Check sheet for the modelled part. Datum: model origin and axes. Units: mm. A direction names the side the tool comes from. Coordinates: 2 decimals unless noted, no trailing zeros. Loops run counter-clockwise (first coordinate to the right, second up) from the corner with the lowest first, then second, coordinate; pieces in that order, holes last. Notation, with made-up numbers: M 66,56.25 L 110,56.25 A18 ccw 110,86.25 Z; hole C 55.5,58.25 d1. An arc over 180 degrees is marked long. Use CSV: the item, a comma, the result in double quotes. Start each with the question number.
(1) Section check C-C on x = 34.5. Record the cut outline in (y, z).
(2) Set-up check for faces 4 (the flat face through (53, -60, 108)), 5 (the flat face through (39, -63, 94)), 6 (the flat face through (26, 1, 94)), 7 (the flat face through (37, -1, 118)): record each of +Z, -Z, +X, -X, +Y, -Y from which the full face is reachable in a straight line by a thin tool's end or side.
(3) Go/stop test with flat-tipped pins: pin 1 Ø8.5 at (y, z) = (-63.5, 114) entering from -X; pin 2 Ø3 at (y, z) = (-1, 115) entering from +X; pin 3 Ø0.9 at (y, z) = (19.5, 118) entering from +X. Record where each tip stops, or that it passes through.
(4) Draft check along Z on faces 1 (the flat face through (20, -1, 99)), 2 (the flat face through (28, -1, 123)), 3 (the flat face through (47, 45, 108)). Enter one of: pulls with the +Z half, pulls with the -Z half, needs draft (parallel to the pull), parting line crosses it, or undercut.
(5) Scan lines: line 1 (Y direction, x = 19.7, z = 99.5); line 2 (Y direction, x = 42, z = 103.25); line 3 (Y direction, x = 41.25, z = 98). Record each from-to range of solid material in increasing order.
(6) Section check B-B on z = 108. Record the cut outline in (x, y), and give its area (3 significant figures).
(7) Section check D-D on y = -57.5. Record the cut outline in (x, z), and give its area (3 significant figures).
(8) Section check A-A on y = -27.5. Record the cut outline in (x, z), and give its area (3 significant figures).
from build123d import *

# Parameters (mm, degrees)
SKETCH003_W             = 30
SKETCH003_H             = 97
PAD002_DEPTH            = 13
SKETCH004_W             = 30
SKETCH004_H             = 6
PAD003_DEPTH            = 15
PAD003_FACE5_W          = 30
PAD003_FACE5_H          = 6
PAD004_DEPTH            = 6
SKETCH005_W             = 28
SKETCH005_H             = 28
PAD005_DEPTH            = 30
SKETCH006_W             = 26
SKETCH006_H             = 26
PAD006_DEPTH            = 1
SKETCH007_W             = 30
SKETCH007_H             = 32
PAD007_DEPTH            = 14
SKETCH008_R             = 1.5
POCKET_DEPTH            = 10
SKETCH009_R             = 3
PAD008_DEPTH            = 85
SKETCH010_W             = 9
SKETCH010_H             = 85
POCKET001_DEPTH         = 4
SKETCH011_R             = 1.5
POCKET002_DEPTH         = 14
SKETCH028_W             = 9.5
SKETCH028_H             = 83
POCKET007_DEPTH         = 12
SKETCH029_W             = 9.5
SKETCH029_H             = 83
POCKET008_DEPTH         = 12
BODY001_PITCH_ANGLE     = -90
BODY001_PLACEMENT_ANGLE = 90


with BuildPart() as part:
    # Sketch003 → Pad002 (new body)
    with BuildSketch(Plane.XZ):
        Rectangle(SKETCH003_W, SKETCH003_H)
    extrude(amount=PAD002_DEPTH)

    # Sketch004 (on Face6 of Pad002) → Pad003 (join)
    with BuildSketch(Plane.XZ.offset(13)):
        with Locations((0, -45.5)):
            Rectangle(SKETCH004_W, SKETCH004_H)
        with Locations((0, 45.5)):
            Rectangle(SKETCH004_W, SKETCH004_H)
    extrude(amount=PAD003_DEPTH)

    # Pad003 Face5 → Pad004 (add)
    with BuildSketch(Plane(origin=(0, -28, 45.5), x_dir=(-1, 0, 0), z_dir=(0, -1, 0))):
        Rectangle(PAD003_FACE5_W, PAD003_FACE5_H)
    extrude(amount=PAD004_DEPTH)

    # Sketch005 (on Face8 of Pad004) → Pad005 (join)
    with BuildSketch(Plane(origin=(0, 0, 48.5), x_dir=(-1, 0, 0), z_dir=(0, 0, 1))):
        with Locations((0, 20)):
            Rectangle(SKETCH005_W, SKETCH005_H)
    extrude(amount=PAD005_DEPTH)

    # Sketch006 (on Face1 of Pad005) → Pad006 (join)
    with BuildSketch(Plane(origin=(0, -13, 10), x_dir=(1, 0, 0), z_dir=(0, -1, 0))):
        with Locations((0, -19.410291)):
            Rectangle(SKETCH006_W, SKETCH006_H)
    extrude(amount=PAD006_DEPTH)

    # Sketch007 (on Face15 of Pad006) → Pad007 (join)
    with BuildSketch(Plane.XZ.offset(14)):
        with Locations((0, -9.410291)):
            Rectangle(SKETCH007_W, SKETCH007_H)
    extrude(amount=PAD007_DEPTH)

    # Sketch008 (on Face24 of Pad007) → Pocket (cut)
    with BuildSketch(Plane.XZ.offset(28)):
        with Locations((-10, 0.589709)):
            Circle(SKETCH008_R)
        with Locations((10, 0.589709)):
            Circle(SKETCH008_R)
        with Locations((10, -19.410291)):
            Circle(SKETCH008_R)
        with Locations((-10, -19.410291)):
            Circle(SKETCH008_R)
    extrude(amount=-POCKET_DEPTH, mode=Mode.SUBTRACT)

    # Sketch009 (on Face5 of Pocket) → Pad008 (join)
    with BuildSketch(Plane(origin=(0, 0, 42.5), x_dir=(1, 0, 0), z_dir=(0, 0, -1))):
        with Locations((0, 20)):
            Circle(SKETCH009_R)
    extrude(amount=PAD008_DEPTH)

    # Sketch010 (on Face1 of Pad008) → Pocket001 (cut)
    with BuildSketch(Plane.XZ.offset(13)):
        Rectangle(SKETCH010_W, SKETCH010_H)
    extrude(amount=-POCKET001_DEPTH, mode=Mode.SUBTRACT)

    # Sketch011 (on Face8 of Pocket001) → Pocket002 (cut)
    with BuildSketch(Plane(origin=(0, 0, 0), x_dir=(1, 0, 0), z_dir=(0, 1, 0))):
        with Locations((-8.5, 27.5)):
            Circle(SKETCH011_R)
        with Locations((8.5, 27.5)):
            Circle(SKETCH011_R)
        with Locations((8.5, -27.5)):
            Circle(SKETCH011_R)
        with Locations((-8.5, -27.5)):
            Circle(SKETCH011_R)
    extrude(amount=-POCKET002_DEPTH, mode=Mode.SUBTRACT)

    # Sketch028 (on Face18 of Pocket002) → Pocket007 (cut)
    with BuildSketch(Plane.XZ.offset(13)):
        with Locations((-9.25, 0)):
            Rectangle(SKETCH028_W, SKETCH028_H)
    extrude(amount=-POCKET007_DEPTH, mode=Mode.SUBTRACT)

    # Sketch029 (on Face1 of Pocket007) → Pocket008 (cut)
    with BuildSketch(Plane.XZ.offset(13)):
        with Locations((9.25, 0)):
            Rectangle(SKETCH029_W, SKETCH029_H)
    extrude(amount=-POCKET008_DEPTH, mode=Mode.SUBTRACT)


with BuildPart() as part_1:
    # Body001 pitch: moved
    add(part.part.rotate(Axis((0, 0, 0), (0, 1, 0)), BODY001_PITCH_ANGLE))


with BuildPart() as part_2:
    # Body001 placement: moved
    add(part_1.part.moved(Location((19, 0, 108))).rotate(Axis((19, 0, 108), (0, 0, 1)), BODY001_PLACEMENT_ANGLE))


solid = part_2.part
Outcome:
1,outline,"M -78.5,94 L -48.5,94 L -48.5,93 L -42.5,93 L -42.5,123 L -48.5,123 L -48.5,122 L -78.5,122 Z; M -6.59,93 L 25.41,93 L 25.41,123 L -6.59,123 Z; M 42.5,93 L 48.5,93 L 48.5,123 L 42.5,123 Z"
2,face 4,"+Z, -Z, +X, +Y, -Y"
2,face 5,"-Z, +X, -X, -Y"
2,face 6,"none"
2,face 7,"+X"
3,pin 1,"stops at x = 25"
3,pin 2,"stops at x = 47"
3,pin 3,"stops at x = 37"
4,face 1,"undercut"
4,face 2,"pulls with the +Z half"
4,face 3,"needs draft"
5,line 1,"y = -48.5 to -29, -26 to 26, 29 to 48.5"
5,line 2,"y = -78.5 to -42.5, -6.59 to 25.41, 42.5 to 48.5"
5,line 3,"y = -78.5 to -42.5, -6.59 to -2.09, 0.91 to 17.91, 20.91 to 25.41, 42.5 to 48.5"
6,outline,"M 19,-48.5 L 25,-48.5 L 25,-78.5 L 53,-78.5 L 53,-42.5 L 42,-42.5 L 42,-6.59 L 47,-6.59 L 47,25.41 L 42,25.41 L 42,42.5 L 47,42.5 L 47,48.5 L 19,48.5 Z; hole M 28,-42.5 L 36,-42.5 L 36,-6.59 L 33,-6.59 L 33,-3.59 L 32,-3.59 L 32,22.41 L 33,22.41 L 33,25.41 L 36,25.41 L 36,42.5 L 28,42.5 Z"
6,area,"2,770 mm²"
7,outline,"M 25,94 L 53,94 L 53,122 L 25,122 Z"
7,area,"784 mm²"
8,outline,"M 19,93 L 32,93 L 32,94 L 20,94 L 20,98 L 19,98 Z; M 19,101 L 20,101 L 20,103.5 L 28,103.5 L 28,112.5 L 20,112.5 L 20,115 L 19,115 Z; M 19,118 L 20,118 L 20,122 L 32,122 L 32,123 L 19,123 Z; C 39,108 d6"
8,area,"148 mm²"
